Here's the drawing with two shaded views (mm, measured from the low corner). I have some questions. Give positions to 0.01 mm unless a question says otherwise; leave off trailing zeros. Write each loop counter-clockwise with the first axis right and the second up, starting at its lowest first coordinate (ties: lowest second). Pieces come first, ordered by that corner, then holes. Notation, with made-up numbers: (-27, 1.25) -> (-1, 1.25) arc R31 ccw to (-1, 29.25) -> close; hole circle Ø1 at (-33.75, 4). An arc over 180 degrees is marked (long way). One line per item, written item: value.
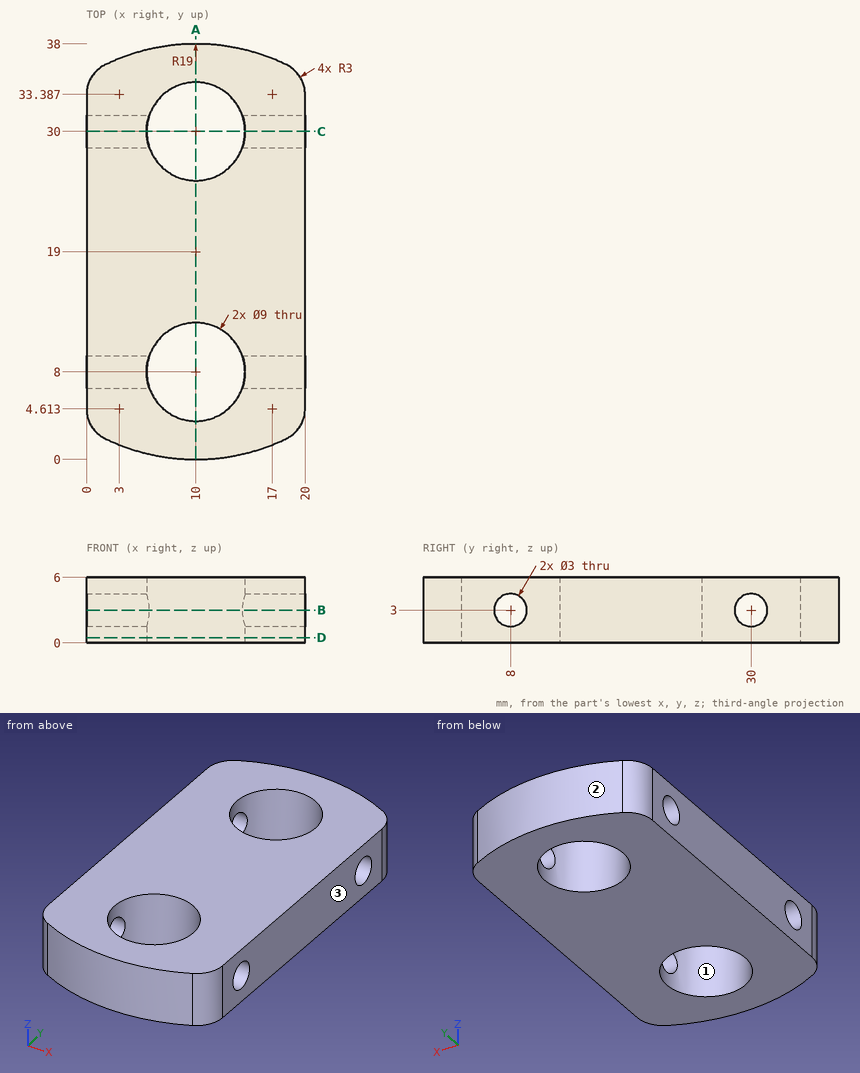
1) If we section it at C-C (y = 30): Write out the boundary of the cut face in (x, z).
Answer list:
outline: (0, 0) -> (5.5, 0) -> (5.5, 1.5) -> (0, 1.5) -> close; (0, 4.5) -> (5.5, 4.5) -> (5.5, 6) -> (0, 6) -> close; (14.5, 0) -> (20, 0) -> (20, 1.5) -> (14.5, 1.5) -> close; (14.5, 4.5) -> (20, 4.5) -> (20, 6) -> (14.5, 6) -> close
2) If we section it at B-B (z = 3): Write out the boundary of the cut face in (x, y) (1 decimal).
Answer list:
outline: (0, 4.6) arc R3 ccw to (1.7, 1.9) arc R19 ccw to (18.3, 1.9) arc R3 ccw to (20, 4.6) -> (20, 6.5) -> (14.2, 6.5) arc R4.5 cw to (5.8, 6.5) -> (0, 6.5) -> close; (0, 9.5) -> (5.8, 9.5) arc R4.5 cw to (14.2, 9.5) -> (20, 9.5) -> (20, 28.5) -> (14.2, 28.5) arc R4.5 cw to (5.8, 28.5) -> (0, 28.5) -> close; (0, 31.5) -> (5.8, 31.5) arc R4.5 cw to (14.2, 31.5) -> (20, 31.5) -> (20, 33.4) arc R3 ccw to (18.3, 36.1) arc R19 ccw to (1.7, 36.1) arc R3 ccw to (0, 33.4) -> close
3) I need wall thicknesses on L1, parallel to Y at x = 10, z = 4; L2, parallel to Y at x = 1.7, z = 3; L3, parallel to Z at x = 16.1, y = 8. Which ranges of each line are inside material? Lowest first, please.
Answer list:
L1: y = 0 to 3.5, 12.5 to 25.5, 34.5 to 38
L2: y = 1.91 to 6.5, 9.5 to 28.5, 31.5 to 36.09
L3: z = 0 to 1.5, 4.5 to 6
4) If we section it at A-A (x = 10): Write out the boundary of the cut face in (y, z), and give its area (3 significant figures).
Answer list:
outline: (0, 0) -> (3.5, 0) -> (3.5, 6) -> (0, 6) -> close; (12.5, 0) -> (25.5, 0) -> (25.5, 6) -> (12.5, 6) -> close; (34.5, 0) -> (38, 0) -> (38, 6) -> (34.5, 6) -> close
area: 120 mm^2
5) If we section it at D-D (z = 0.5): Write out the boundary of the cut face in (x, y) (1 decimal), and give its area (3 significant figures).
Answer list:
outline: (0, 4.6) arc R3 ccw to (1.7, 1.9) arc R19 ccw to (18.3, 1.9) arc R3 ccw to (20, 4.6) -> (20, 33.4) arc R3 ccw to (18.3, 36.1) arc R19 ccw to (1.7, 36.1) arc R3 ccw to (0, 33.4) -> close; hole circle Ø9 at (10, 8); hole circle Ø9 at (10, 30)
area: 594 mm^2
6) We'd pull the mould along X, two halves only. Please class the marked faces 1, 2 and 3: released by +X, released by -X, zero draft, split by the parting line, or undercut.
Answer list:
face 1: undercut
face 2: split by the parting line
face 3: released by +X
